Work out the finished part from the listing and answer in its coordinate system (mm). A direction names the side the tool comes from. Round coordinates to 2 decimals unless told otherwise and drop trailing zeros.
1. Straight lines are drawn through the part: probe 1 along Z at (x, y) = (0.6, -17.5); probe 2 along Y at (x, z) = (2.5, 0.75); probe 3 along Y at (x, z) = (-0.5, 0.5). For each, find the intervals that lie inside material, in ascending order.
2. Flat-ended cylindrical pins translate along their axes: pin 1 Ø1.4 at (y, z) = (-17.5, 0) entering from +X; pin 2 Ø3 at (x, y) = (0.5, 96) entering from +Z; pin 3 Ø2 at (x, y) = (-2, 172) entering from +Z. Find the tip coordinate at first contact, or state that the pin passes through.
3. A tool of negligible diameter and unlimited length cuts with its end or side. For faces 1 (the face through (-2.44, 202.46, -0.54)), 2 (the face through (2, 0, 2)), 3 (the face through (-3.417, 194.93, -0.759)), 4 (the face through (-2.44, -12.54, 0.54)), from which of +Z, -Z, +X, -X, +Y, -Y can it reach the whole face along a straight path? Write none if from no direction.
4. Determine the mould class of faces 5 (the face through (-2, 200, 2)), 6 (the face through (3.417, -5.07, -0.759)), 7 (the face through (-2.44, 93.67, -0.54)) for opening direction Y: pulls with the +Y half, pulls with the -Y half, needs draft (parallel to the pull), parting line crosses it, or undercut.
```python
from build123d import *

# Parameters (mm, degrees)
CROQUIS1_R               = 2.5
SALIENTE_EXTRUIR6_DEPTH  = 190
CROQUIS4_R               = 3.5
SALIENTE_EXTRUIR7_DEPTH  = 10
CROQUIS5_R               = 2.5
SALIENTE_EXTRUIR9_DEPTH  = 5
SALIENTE_EXTRUIR10_START = 10
CROQUIS6_R               = 3.5
SALIENTE_EXTRUIR10_DEPTH = 10
SALIENTE_EXTRUIR11_START = 5
CROQUIS7_R               = 2.5
SALIENTE_EXTRUIR11_DEPTH = 5
SALIENTE_EXTRUIR12_DEPTH = 1
CROQUIS10_R              = 0.6
CORTAR_EXTRUIR1_DEPTH    = 12.5
REDONDEO3_R              = 1
REDONDEO4_R              = 1


with BuildPart() as part:
    # Croquis1 → Saliente-Extruir6 (new body)
    with BuildSketch(Plane(origin=(0, 0, 0), x_dir=(1, 0, 0), z_dir=(0, 1, 0))):
        with Locations(Location((0, 0, 0), (0, 0, 270))):
            Circle(CROQUIS1_R)
    extrude(amount=SALIENTE_EXTRUIR6_DEPTH)

    # Croquis4 → Saliente-Extruir7 (add)
    with BuildSketch(Plane(origin=(0, 190, 0), x_dir=(1, 0, 0), z_dir=(0, 1, 0))):
        with Locations(Location((0, 0, 0), (0, 0, 270))):
            Circle(CROQUIS4_R)
    extrude(amount=SALIENTE_EXTRUIR7_DEPTH)

    # Croquis5 → Saliente-Extruir9 (add)
    with BuildSketch(Plane(origin=(0, 200, 0), x_dir=(1, 0, 0), z_dir=(0, 1, 0))):
        with Locations(Location((0, 0, 0), (0, 0, 270))):
            Circle(CROQUIS5_R)
    extrude(amount=SALIENTE_EXTRUIR9_DEPTH)

    # Croquis6 → Saliente-Extruir10 (add)
    with BuildSketch(Plane.XZ.offset(SALIENTE_EXTRUIR10_START)):
        with Locations(Location((0, 0, 0), (0, 0, 90))):
            Circle(CROQUIS6_R)
    extrude(amount=-SALIENTE_EXTRUIR10_DEPTH)

    # Croquis7 → Saliente-Extruir11 (add)
    with BuildSketch(Plane.XZ.offset(10).offset(SALIENTE_EXTRUIR11_START)):
        with Locations(Location((0, 0, 0), (0, 0, 270))):
            Circle(CROQUIS7_R)
    extrude(amount=-SALIENTE_EXTRUIR11_DEPTH)

    # Croquis8 → Saliente-Extruir12 (add, symmetric)
    with BuildSketch(Plane.XY):
        Polygon((1, 210), (-1, 210), (-1, 205), (0, 205), (1, 205), align=None)
        Polygon((0, -15), (1, -15), (1, -20), (-1, -20), (-1, -15), align=None)
    extrude(amount=SALIENTE_EXTRUIR12_DEPTH, both=True)

    # Croquis10 → Cortar-Extruir1 (cut, symmetric)
    with BuildSketch(Plane(origin=(0, 0, 0), x_dir=(0, 0, -1), z_dir=(1, 0, 0))):
        with Locations((0, -17.5)):
            Circle(CROQUIS10_R)
        with Locations(Location((0, 207.5, 0), (0, 0, 90))):
            Circle(CROQUIS10_R)
    extrude(amount=CORTAR_EXTRUIR1_DEPTH, both=True, mode=Mode.SUBTRACT)

    # Redondeo3
    redondeo3_edges = [part.edges().sort_by_distance(p)[0] for p in [
        (0, -20, 1),
    ]]
    fillet(redondeo3_edges, radius=REDONDEO3_R)

    # Redondeo4
    redondeo4_edges = [part.edges().sort_by_distance(p)[0] for p in [
        (0, 210, 1),
        (0, 210, -1),
        (0, -20, -1),
    ]]
    fillet(redondeo4_edges, radius=REDONDEO4_R - 0.0001)  # a hair under: the kernel refuses the full size


solid = part.part
```
Worked answers:
1. probe 1: z = -1 to -0.6, 0.6 to 1
1. probe 2: y = -10 to 0, 190 to 200
1. probe 3: y = -19.87 to -17.83, -17.17 to 207.17, 207.83 to 209.87
2. pin 1: stops at x = 1
2. pin 2: stops at z = 2.5
2. pin 3: stops at z = 2.29
3. face 1: +Y
3. face 2: none
3. face 3: +Y, -Y
3. face 4: -Y
4. face 5: pulls with the +Y half
4. face 6: needs draft
4. face 7: undercut
